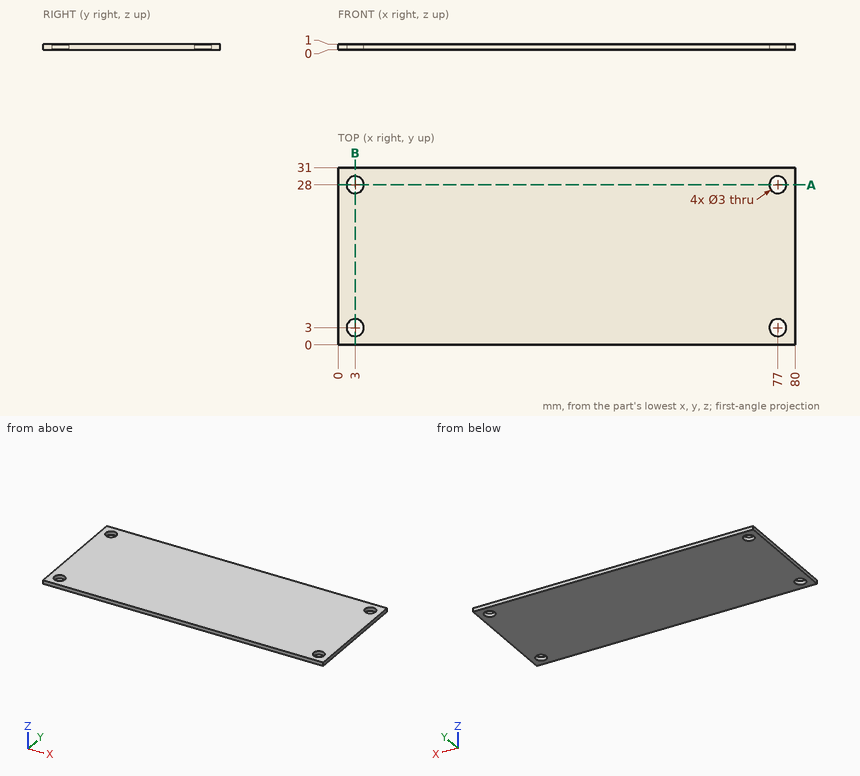
For this review, use the dimensioned drawing (mm, ordinates from the lowest corner) and the shaded views. Round coordinates to 2 decimals unless told otherwise and drop trailing zeros. Order: outer loops, then holes, each group sorted by start corner. A loop starts at its lowest first (then second) coordinate and runs counter-clockwise, first axis right, second up. Notation, with made-up numbers: (48, 7.25) - (93, 7.25) arc R36 cw to (93, 45.25) - close; hole circle Ø11 at (7, 58). An arc over 180 degrees is marked (long way). Use one line per item in the form item = value.
Q1. Add section A-A on y = 28. Give the boundary of the cut face in (x, z), then the cut area to 3 significant figures.
Response values:
outline = (0, 0) - (1.5, 0) - (1.5, 1) - (0, 1) - close; (4.5, 0) - (75.5, 0) - (75.5, 1) - (4.5, 1) - close; (78.5, 0) - (80, 0) - (80, 1) - (78.5, 1) - close
area = 74.0 mm^2
Q2. Clearance check with a flat-ended pin moving along its axis: P1, Ø5, axis at x = 12.5, y = 7, coming from the -Z side. State where the tip first meets the part, or that it passes through.
Response values:
P1 = 0
Q3. Add section B-B on x = 3. Give the boundary of the cut face in (y, z).
Response values:
outline = (0, 0) - (1.5, 0) - (1.5, 1) - (0, 1) - close; (4.5, 0) - (26.5, 0) - (26.5, 1) - (4.5, 1) - close; (29.5, 0) - (31, 0) - (31, 1) - (29.5, 1) - close
Q4. To check wall thickness, follow line 1 (Y direction, x = 77, z = 0.7); line 2 (X direction, y = 3.5, z = 0.7); line 3 (X direction, y = 4, z = 0.3). State the ranges of each line that lie inside material, in increasing order.
Response values:
line_1 = 0 to 1.5, 4.5 to 26.5, 29.5 to 31
line_2 = 0 to 1.59, 4.41 to 75.59, 78.41 to 80
line_3 = 0 to 1.88, 4.12 to 75.88, 78.12 to 80
